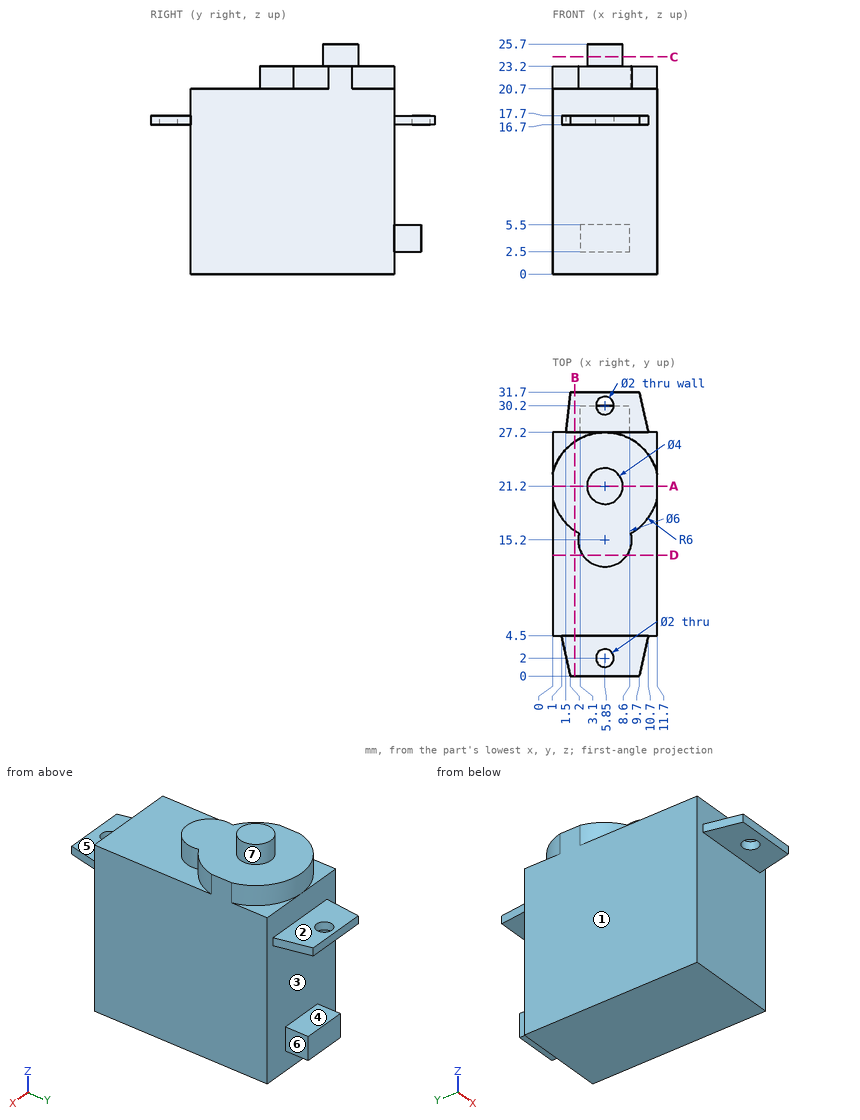
Part print with two shaded views. Sizes in mm from the minimum x, y, z corner. A direction names the side the tool comes from. Give positions to 0.01 mm unless a question says otherwise; leave off trailing zeros. Order: outer loops, then holes, each group sorted by start corner. A loop starts at its lowest first (then second) coordinate and runs counter-clockwise, first axis right, second up.
1) Saw through at C-C, the plane z = 24.25. Write the cut outline in (x, y), then the cut area to 3 significant figures.
2) Pin check, flat tips, straight feed: pin 1 (1.4 mm diameter, centred on x = 9.5, y = 24, fed in from +Z); pin 2 (2.5 mm diameter, centred on x = 6, y = 30, fed in from +Z); pin 3 (6 mm diameter, centred on x = 4.5, z = 8.5, fed in from -Y). Stop position of each tip, or through.
3) Mould opens along Z. For the marked faces 1, 2, 3 and 4 say: +Z half, -Z half, draft (parallel to the pull), parting line (faces both ways), or undercut.
4) 3-axis set-ups, long thin cutter, end or side, ignore diameter. For the marked faces 5, 6 and 7: which of +Z, -Z, +X, -X, +Y, -Y reach the whole face in a straight line?
5) Saw through at A-A, the plane y = 21.2. Write the cut outline in (x, z).
6) Wall check: probe 1 along Y at (x, z) = (5.85, 17.3); probe 2 along Z at (x, y) = (8, 27.5); probe 3 along Y at (x, z) = (6.25, 11.5). Give the ranges that are in metal, low to high.
7) Saw through at B-B, the plane x = 2.5. Write the cut outline in (y, z).
8) Saw through at D-D, the plane y = 13.5. Write the cut outline in (x, z).
Computed:
1. outline: circle Ø4 at (5.85, 21.2)
1. area: 12.6 mm2
2. pin 1: stops at z = 23.2
2. pin 2: stops at z = 17.7
2. pin 3: stops at y = 4.5
3. face 1: draft
3. face 2: +Z half
3. face 3: undercut
3. face 4: undercut
4. face 5: +Z, +X, -X, -Y
4. face 6: -Z, +X, +Y
4. face 7: +Z
5. outline: (0, 0) - (11.7, 0) - (11.7, 23.2) - (7.85, 23.2) - (7.85, 25.7) - (3.85, 25.7) - (3.85, 23.2) - (0, 23.2) - close
6. probe 1: y = 0 to 1, 3 to 29.2, 31.2 to 31.7
6. probe 2: z = 2.5 to 5.5, 16.7 to 17.7
6. probe 3: y = 4.5 to 27.2
7. outline: (0, 16.7) - (4.5, 16.7) - (4.5, 0) - (27.2, 0) - (27.2, 16.7) - (31.7, 16.7) - (31.7, 17.7) - (27.2, 17.7) - (27.2, 20.7) - (26.18, 20.7) - (26.18, 23.2) - (16.22, 23.2) - (16.22, 20.7) - (4.5, 20.7) - (4.5, 17.7) - (0, 17.7) - close
8. outline: (0, 0) - (11.7, 0) - (11.7, 20.7) - (8.32, 20.7) - (8.32, 23.2) - (3.38, 23.2) - (3.38, 20.7) - (0, 20.7) - close
